Could you check a few things on this model? Use its own coordinates, in mm. A direction names the side the tool comes from. Round coordinates to 2 decimals unless told otherwise and drop trailing zeros. Loops run counter-clockwise (first coordinate to the right, second up) from the corner with the lowest first, then second, coordinate; pieces in that order, holes last. Notation, with made-up numbers: (42, 56.5) -> (90, 56.5) arc R34 cw to (90, 93.5) -> close; hole circle Ø9 at (-18.5, 12.5). An arc over 180 degrees is marked (long way). Write each question's results on one line, items separated by ' | '. Start each with the question number.
1) Imagine slicing it at A-A, the plane z = 10.5. List the corners of the cut face in (x, y) for me, plus the area to 4 significant figures.
2) If I drill on probe 1 along Z at (x, y) = (-21, 3.5); probe 2 along Z at (x, y) = (-2, 36); probe 3 along Y at (x, z) = (21, 16.75), over which ranges is the centre line in solid material (lowest first)?
3) Imagine slicing it at D-D, the plane y = -4.5. Give the number of separate pieces and of enclosed holes in the cut face, plus the area to 3 significant figures.
4) Which directions (+Z, -Z, +X, -X, +Y, -Y) give clear straight access to the entire face, cutting with the end or side of a thin tool? Please do faces 4 (the flat face through (19.774, -2.999, 10.938)), 5 (the flat face through (22.966, 1.494, 10.07)), 6 (the flat face through (7.07, -18.71, 2.54)), 7 (the flat face through (-22.966, -1.494, 10.07)).
5) Imagine slicing it at B-B, the plane x = -16.5. List the corners of the cut face in (y, z) for me.
6) For P1, Ø8, axis at x = 26.96, y = -21.09, coming from the +Z side; P2, Ø8, axis at y = 8.5, z = 5.5, coming from the -X side, each with a flat end and sliding along its axis, tell me the tip position at first contact or that it passes through.
7) Imagine slicing it at C-C, the plane y = 19.5. List the corners of the cut face in (x, z) for me.
8) We'd pull the mould along Z, two halves only. Please class faces 1 (the cylindrical face through (22.18, -3.56, 20)), 2 (the flat face through (-24.715, 3.766, 10.938)), 3 (the cylindrical face through (-22.022, 4.587, 12.782)): pulls with the +Z half, pulls with the -Z half, needs draft (parallel to the pull), parting line crosses it, or undercut.
from build123d import *

# Parameters (mm, degrees)
F1_DEPTH  = 5
F2_R      = 2.5
F3_DEPTH  = 25
F5_DEPTH  = 6
F7_DEPTH  = 5
F8_R      = 2.5
F9_DEPTH  = 25
F10_R     = 2.5
F11_DEPTH = 5


with BuildPart() as f1:
    # F0 (on Top) → F1 (new body)
    with BuildSketch(Plane.XY):
        Polygon((31.50713, -24.643473), (37.095438, 14.964239), (5.588308, 39.607712), (-31.50713, 24.643473), (-37.095438, -14.964239), (-5.588308, -39.607712), align=None)
    extrude(amount=F1_DEPTH)

    # F2 (on face) → F3 (cut)
    with BuildSketch(Plane(origin=(0, 0, 0), x_dir=(1, 0, 0), z_dir=(0, 0, -1))):
        with Locations((31.741173, -12.804337)):
            Circle(F2_R)
        with Locations((4.781705, -33.890831)):
            Circle(F2_R)
        with Locations((-26.959468, -21.086494)):
            Circle(F2_R)
        with Locations((-31.741173, 12.804337)):
            Circle(F2_R)
        with Locations((-4.781705, 33.890831)):
            Circle(F2_R)
        with Locations((26.959468, 21.086494)):
            Circle(F2_R)
    extrude(amount=-F3_DEPTH, mode=Mode.SUBTRACT)

    # F4 (on face) → F5 (cut)
    with BuildSketch(Plane.XY.offset(5)):
        Polygon((17.991608, -14.47879), (21.534804, 8.341794), (3.543196, 22.820585), (-17.991608, 14.47879), (-21.534804, -8.341794), (-3.543196, -22.820585), align=None)
    extrude(amount=-F5_DEPTH, mode=Mode.SUBTRACT)

    # F6 (on face) → F7 (join)
    with BuildSketch(Plane(origin=(-19.763206, 3.068498, 0), x_dir=(0.153425, 0.98816, 0), z_dir=(0.98816, -0.153425, 0))):
        with BuildLine():
            Line((-5, 15), (-5, 5))
            Line((-5, 5), (5, 5))
            Line((5, 5), (5, 15))
            ThreePointArc((5, 15), (0, 20), (-5, 15))
        make_face()
    extrude(amount=-F7_DEPTH)

    # F8 (on face) → F9 (cut)
    with BuildSketch(Plane(origin=(-19.763206, 3.068498, 0), x_dir=(0.153425, 0.98816, 0), z_dir=(0.98816, -0.153425, 0))):
        with Locations((0, 15)):
            Circle(F8_R)
    extrude(amount=-F9_DEPTH, mode=Mode.SUBTRACT)

    # F10 (on face) → F11 (join)
    with BuildSketch(Plane(origin=(19.763206, -3.068498, 0), x_dir=(-0.153425, -0.98816, 0), z_dir=(-0.98816, 0.153425, 0))):
        with BuildLine():
            Line((-5, 15), (-5, 5))
            Line((-5, 5), (5, 5))
            Line((5, 5), (5, 15))
            ThreePointArc((5, 15), (0, 20), (-5, 15))
        make_face()
        with Locations((0, 15)):
            Circle(F10_R, mode=Mode.SUBTRACT)
    extrude(amount=-F11_DEPTH)


solid = f1.part
Checked values:
1) outline: (-25.47, -1.11) -> (-20.53, -1.87) -> (-19, 8.01) -> (-23.94, 8.78) -> close; (19, -8.01) -> (23.94, -8.78) -> (25.47, 1.11) -> (20.53, 1.87) -> close | area: 100.0 mm^2
2) probe 1: 0 to 12.51, 17.49 to 19.99 | probe 2: 0 to 5 | probe 3: -8 to -5.07, -1.45 to 1.48
3) separate pieces: 3 | enclosed holes: 0 | area: 200 mm^2
4) face 4: +Z, -Z, +Y | face 5: +Z, +X, +Y | face 6: +Z, -Z | face 7: +Z, -X, -Y
5) outline: (-31.07, 0) -> (-12.39, 0) -> (-12.39, 5) -> (-31.07, 5) -> close; (15.06, 0) -> (30.7, 0) -> (30.7, 5) -> (15.06, 5) -> close
6) P1: z = 5 | P2: x = -34.34
7) outline: (-32.23, 0) -> (-28.89, 0) -> (-28.89, 5) -> (-32.23, 5) -> close; (-25.03, 0) -> (-5.03, 0) -> (-5.03, 5) -> (-25.03, 5) -> close; (7.67, 0) -> (31.3, 0) -> (31.3, 5) -> (7.67, 5) -> close
8) face 1: pulls with the +Z half | face 2: needs draft | face 3: undercut
